Check sheet for the drawn part. Datum: minimum x, y, z corner. Units: mm. A direction names the side the tool comes from. Coordinates: 2 decimals unless noted, no trailing zeros. Write each loop counter-clockwise with the first axis right and the second up, starting at its lowest first coordinate (ties: lowest second). Pieces come first, ordered by that corner, then holes. Notation, with made-up numbers: (33, 40) -> (78, 40) arc R31 cw to (78, 67) -> close; hole circle Ø8 at (-14.5, 72.25). An arc over 180 degrees is marked (long way). One line per question, with ' | ' between items.
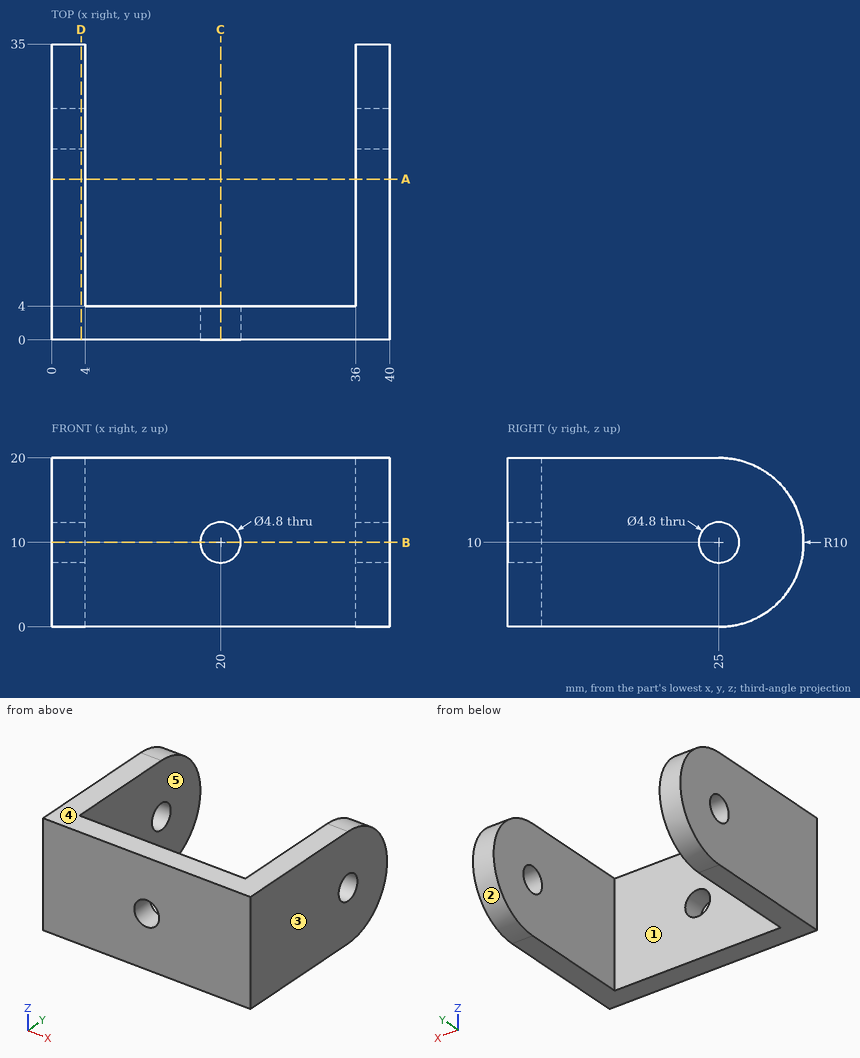
1. Go/stop test with flat-tipped pins: P1, Ø4.5, axis at y = 25, z = 10, coming from the -X side; P2, Ø10, axis at x = 17, z = 8.5, coming from the +Y side. Record where each tip stops, or that it passes through.
Worked answers:
P1: through | P2: y = 4
2. Cross-section at C-C on x = 20. Record the boundary of the cut face in (y, z).
Worked answers:
outline: (0, 0) -> (4, 0) -> (4, 7.6) -> (0, 7.6) -> close; (0, 12.4) -> (4, 12.4) -> (4, 20) -> (0, 20) -> close
3. Tool access check on the marked faces 4 and 5. Record the directions out of +Z, -Z, +X, -X, +Y, -Y that give a thin tool (end or side, any length) a straight path to the whole face; none if there is none.
Worked answers:
face 4: +Z, +X, -X, +Y, -Y | face 5: +Z, -Z, +Y
4. Material ranges on line 1 (Z direction, x = 20, y = 0.9); line 2 (X direction, y = 30, z = 4); line 3 (X direction, y = 2.6, z = 10), recorded low to high. Write a range as from..to.
Worked answers:
line 1: 0..7.6, 12.4..20 | line 2: 0..4, 36..40 | line 3: 0..17.6, 22.4..40
5. Mould release check, pull along X, two halves, no side actions. Record for the marked faces 1, 2 and 3: released by +X, released by -X, zero draft, split by the parting line, or undercut.
Worked answers:
face 1: undercut | face 2: zero draft | face 3: released by +X
6. Cross-section at A-A on y = 19. Record the boundary of the cut face in (x, z).
Worked answers:
outline: (0, 0) -> (4, 0) -> (4, 20) -> (0, 20) -> close; (36, 0) -> (40, 0) -> (40, 20) -> (36, 20) -> close
7. Cross-section at D-D on x = 3.5. Record the boundary of the cut face in (y, z).
Worked answers:
outline: (0, 0) -> (25, 0) arc R10 ccw to (25, 20) -> (0, 20) -> close; hole circle Ø4.8 at (25, 10)
8. Cross-section at B-B on z = 10. Record the boundary of the cut face in (x, y).
Worked answers:
outline: (0, 0) -> (17.6, 0) -> (17.6, 4) -> (4, 4) -> (4, 22.6) -> (0, 22.6) -> close; (0, 27.4) -> (4, 27.4) -> (4, 35) -> (0, 35) -> close; (22.4, 0) -> (40, 0) -> (40, 22.6) -> (36, 22.6) -> (36, 4) -> (22.4, 4) -> close; (36, 27.4) -> (40, 27.4) -> (40, 35) -> (36, 35) -> close
